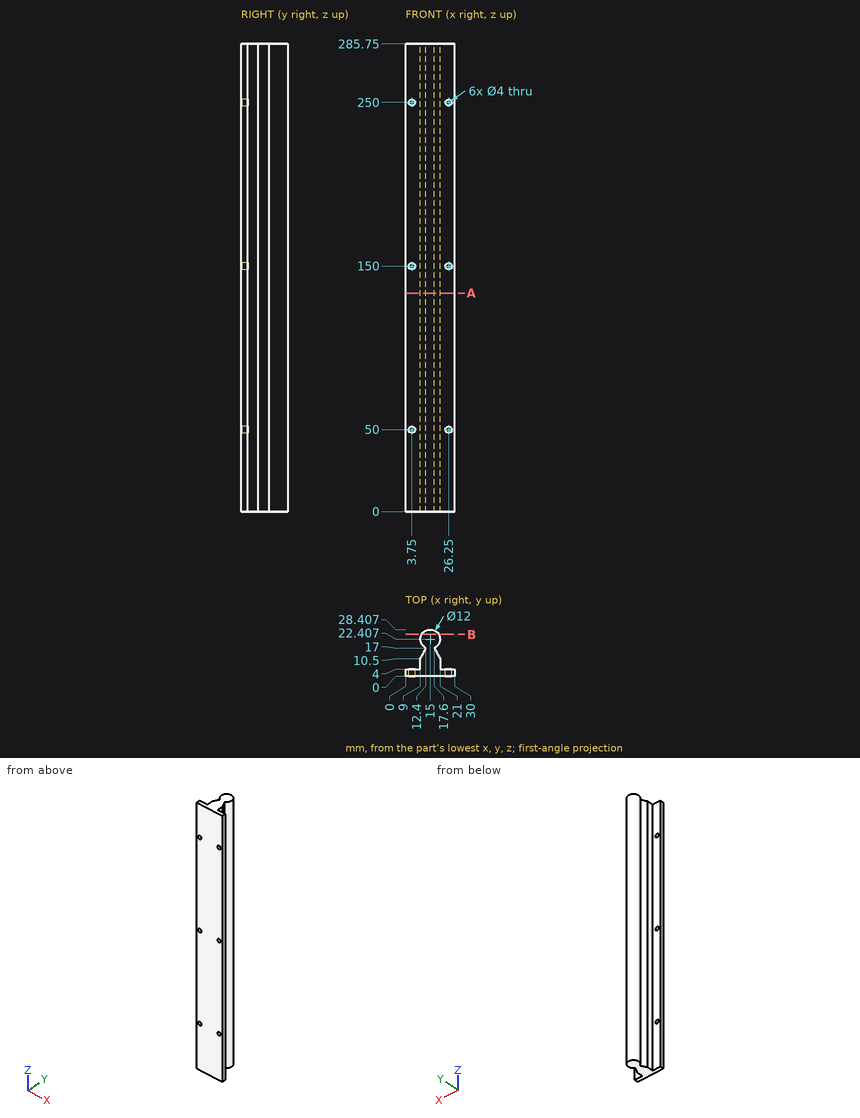
Print and shaded views of the part. All mm, measured from the part's lowest x, y and z. Coordinates: 2 decimals unless noted, no trailing zeros. Write each loop counter-clockwise with the first axis right and the second up, starting at its lowest first coordinate (ties: lowest second). Pieces come first, ordered by that corner, then holes. Notation, with made-up numbers: M -33.75,-21 L 0.25,-21 A17 cw 0.25,8 Z; hole C 66,-21 d11. An arc over 180 degrees is marked long. Return JSON: item names as keys, results as strings.
1. Flat gauge pins, fed straight in: pin 1 Ø1.5 at (x, y) = (23.5, 6.5) entering from -Z; pin 2 Ø10 at (x, y) = (11, 14.5) entering from -Z; pin 3 Ø4.5 at (x, z) = (26.25, 250) entering from +Y; pin 4 Ø7 at (x, z) = (23.5, 195) entering from +Y (1 decimal). Where does each tip first touch, or does it go through?
Determined:
{"pin 1": "through", "pin 2": "z = 0", "pin 3": "y = 4", "pin 4": "y = 25.7"}
2. Saw through at A-A, the plane z = 133.5. Write the cut outline in (x, y).
Determined:
{"outline": "M 0,0 L 30,0 L 30,4 L 21,4 L 21,10.5 L 17.6,17 A6 ccw long 12.4,17 L 9,10.5 L 9,4 L 0,4 Z"}
3. Saw through at B-B, the plane y = 25.5. Write the cut outline in (x, z), then the cut area to 3 significant figures.
Determined:
{"outline": "M 9.86,0 L 20.14,0 L 20.14,285.75 L 9.86,285.75 Z", "area": "2,940 mm²"}
4. Probe L1, parallel to X at y = 2.35, z = 250; L2, parallel to Y at x = 4.25, z = 60.5; L3, parallel to Y at x = 14.75, z = 147. List the from-to ranges inside material, lowest first.
Determined:
{"L1": "0 to 1.75, 5.75 to 24.25, 28.25 to 30", "L2": "0 to 4", "L3": "0 to 28.4"}
